Verification items for this drawing (mm, ordinates from the low corner). A direction names the side the tool comes from. Coordinates: 2 decimals unless noted, no trailing zeros. Write each loop counter-clockwise with the first axis right and the second up, starting at its lowest first coordinate (ties: lowest second). Pieces come first, ordered by that corner, then holes. Notation, with made-up numbers: (3.5, 33.5) -> (44.5, 33.5) arc R17 cw to (44.5, 52.5) -> close; hole circle Ø9 at (76, 61.25). An arc over 180 degrees is marked (long way). One line per item, written item: value. Start each with the question number.
1) Set-up check for the marked faces 4, 5, 6, 7 and 8: record each of +Z, -Z, +X, -X, +Y, -Y from which the full face is reachable in a straight line by a thin tool's end or side.
2) Sectioned sample at B-B on z = 32. Enter the section's corners in (x, y), plus the area to 3 significant figures.
3) Gauge pin test, flat ends, axial feed: P1, Ø6, axis at y = 45.5, z = 33.5, coming from the -X side; P2, Ø4, axis at y = 4.5, z = 29.5, coming from the +X side; P3, Ø3, axis at x = 66, z = 20, coming from the -Y side. Record the tip position at first contact, or that the pin passes through.
4) Sectioned sample at C-C on x = 52. Enter the section's corners in (y, z) (1 decimal), plus the area to 3 significant figures.
5) Sectioned sample at A-A on y = 26.5. Enter the section's corners in (x, z).
6) Draft check along Y on the marked faces 1, 2 and 3. Enter one of: +Y half, -Y half, draft (parallel to the pull), parting line (faces both ways), or undercut.
7) Scan lines: line 1 along X through (y, z) = (16.5, 44); line 2 along Z through (x, y) = (50, 41.5) (1 decimal); line 3 along X through (y, z) = (45, 14). Record each from-to range of solid material in increasing order. Write a range as [from, to].
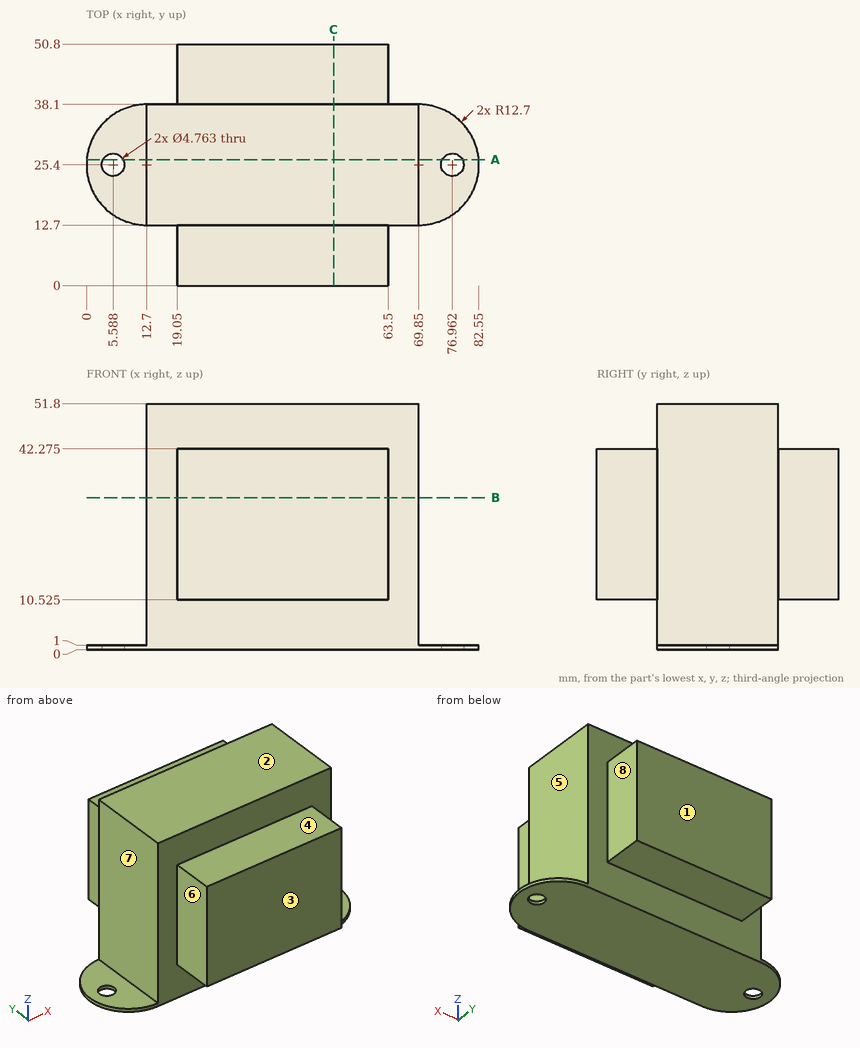
Answers:
1. face 4: +Z, +X, -X, -Y
1. face 5: +Z, +X, +Y, -Y
1. face 6: +Z, -Z, -X, -Y
1. face 7: +Z, -X, +Y, -Y
1. face 8: +Z, -Z, +X, +Y
2. outline: (12.7, 12.7) -> (19.05, 12.7) -> (19.05, 0) -> (63.5, 0) -> (63.5, 12.7) -> (69.85, 12.7) -> (69.85, 38.1) -> (63.5, 38.1) -> (63.5, 50.8) -> (19.05, 50.8) -> (19.05, 38.1) -> (12.7, 38.1) -> close
2. area: 2,580 mm2
3. P1: stops at x = 19.05
3. P2: stops at x = 63.5
3. P3: stops at y = 12.7
4. outline: (0, 10.5) -> (12.7, 10.5) -> (12.7, 0) -> (38.1, 0) -> (38.1, 10.5) -> (50.8, 10.5) -> (50.8, 42.3) -> (38.1, 42.3) -> (38.1, 51.8) -> (12.7, 51.8) -> (12.7, 42.3) -> (0, 42.3) -> close
4. area: 2,120 mm2
5. outline: (0.05, 0) -> (3.48, 0) -> (3.48, 1) -> (0.05, 1) -> close; (7.7, 0) -> (74.85, 0) -> (74.85, 1) -> (69.85, 1) -> (69.85, 51.8) -> (12.7, 51.8) -> (12.7, 1) -> (7.7, 1) -> close; (79.07, 0) -> (82.5, 0) -> (82.5, 1) -> (79.07, 1) -> close
6. face 1: +Y half
6. face 2: draft
6. face 3: -Y half
7. line 1: x = [12.7, 69.85]
7. line 2: z = [10.5, 42.3]
7. line 3: x = [19.05, 63.5]
